For this review, use the dimensioned drawing (mm, ordinates from the lowest corner) and the shaded views. A direction names the side the tool comes from. Round coordinates to 2 decimals unless told otherwise and drop trailing zeros. Write each loop counter-clockwise with the first axis right and the second up, starting at its lowest first coordinate (ties: lowest second). Pieces come first, ordered by that corner, then holes. Notation, with made-up numbers: M 41,80 L 49,80 A18 ccw 49,109 Z; hole C 28.5,-24.75 d3. An arc over 180 degrees is marked long. Answer in a Markdown table with one row per item.
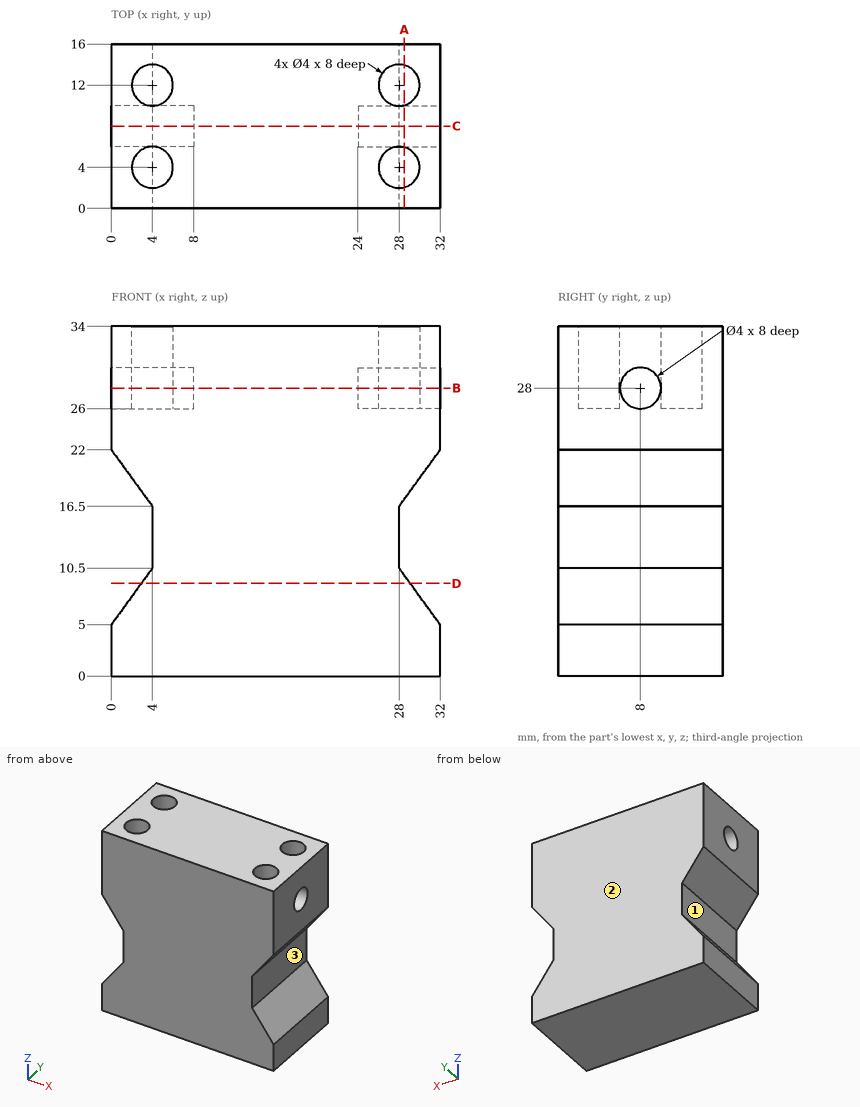
Q1. Take a section at C-C (y = 8). State the section outline as (x, z) points, then the cut area to 3 significant figures.
Found:
| item | result |
|---|---|
| outline | M 0,0 L 32,0 L 32,5 L 28,10.5 L 28,16.5 L 32,22 L 32,26 L 24,26 L 24,30 L 32,30 L 32,34 L 0,34 L 0,30 L 8,30 L 8,26 L 0,26 L 0,22 L 4,16.5 L 4,10.5 L 0,5 Z |
| area | 932 mm² |
Q2. Take a section at A-A (x = 28.5). State the section outline as (y, z) points, then the cut area to 3 significant figures.
Found:
| item | result |
|---|---|
| outline | M 0,0 L 16,0 L 16,9.81 L 0,9.81 Z; M 0,17.19 L 16,17.19 L 16,34 L 13.94,34 L 13.94,26 L 10.06,26 L 10.06,34 L 5.94,34 L 5.94,26 L 2.06,26 L 2.06,34 L 0,34 Z; hole C 8,28 d4 |
| area | 351 mm² |
Q3. Machinability: for the marked faces 1, 2 and 3, which of the approach directions +Z, -Z, +X, -X, +Y, -Y give a long, thin tool a straight path to every point of the face, cutting with its end or side? Answer none if there is none.
Found:
| item | result |
|---|---|
| face 1 | -X, +Y, -Y |
| face 2 | +Z, -Z, +X, -X, +Y |
| face 3 | +X, +Y, -Y |
Q4. For probe 1 along Y at (x, z) = (28, 30.75); probe 2 along X at (y, z) = (12, 30); probe 3 along Y at (x, z) = (28, 29.75), list the stretches that pass through material, from the lowest coordinate up.
Found:
| item | result |
|---|---|
| probe 1 | 0 to 2, 6 to 10, 14 to 16 |
| probe 2 | 0 to 2, 6 to 26, 30 to 32 |
| probe 3 | 0 to 2, 6 to 7.03, 8.97 to 10, 14 to 16 |
Q5. Take a section at D-D (z = 9). State the section outline as (x, y) points.
Found:
| item | result |
|---|---|
| outline | M 2.91,0 L 29.09,0 L 29.09,16 L 2.91,16 Z |
Q6. Take a section at B-B (z = 28). State the section outline as (x, y) points.
Found:
| item | result |
|---|---|
| outline | M 0,0 L 32,0 L 32,6 L 24,6 L 24,10 L 32,10 L 32,16 L 0,16 L 0,10 L 8,10 L 8,6 L 0,6 Z; hole C 4,4 d4; hole C 4,12 d4; hole C 28,4 d4; hole C 28,12 d4 |
Q7. Insertion check: P1, Ø1.2, axis at x = 27.5, y = 4.5, coming from the +Z side; P2, Ø3.5, axis at y = 8, z = 28, coming from the -X side; P3, Ø5, axis at y = 6, z = 12.5, coming from the +X side. Each pin has a flat end and moves straight along its axis. Give the tip position at first contact, or say it passes through.
Found:
| item | result |
|---|---|
| P1 | z = 26 |
| P2 | x = 8 |
| P3 | x = 28.36 |
